Geometry check sheet. Reference: the model listing, model coordinates, mm. Face numbers are marked on the shaded views. A direction names the side the tool comes from. Give positions to 0.01 mm unless a question says otherwise; leave off trailing zeros. Write each loop counter-clockwise with the first axis right and the second up, starting at its lowest first coordinate (ties: lowest second). Pieces come first, ordered by that corner, then holes. Notation, with made-up numbers: M 1,54.5 L 38,54.5 A21 ccw 38,82.5 Z; hole C 12.5,50.25 d9. An arc over 180 degrees is marked long. Write each question's results on one line, items separated by ' | '.
```python
from build123d import *

# Parameters (mm, degrees)
BOSS_EXTRU_1_DEPTH      = 3
BOSS_EXTRU_2_START      = -3
ESQUISSE2_W             = 33.166247904
ESQUISSE2_H             = 3
BOSS_EXTRU_2_DEPTH      = 10
ENL_V_MAT_EXTRU_1_DEPTH = 10
ESQUISSE4_R             = 1.5
ENL_V_MAT_EXTRU_2_DEPTH = 10
ESQUISSE5_R             = 1
ENL_V_MAT_EXTRU_3_DEPTH = 44.588989435
ENL_V_MAT_EXTRU_4_DEPTH = 45.373415465
ESQUISSE7_R             = 1.5
ENL_V_MAT_EXTRU_5_DEPTH = 45.373415465
ESQUISSE8_R             = 1
ENL_V_MAT_EXTRU_6_DEPTH = 3


with BuildPart() as part:
    # Esquisse1 → Boss.-Extru.1 (new body)
    with BuildSketch(Plane.XY):
        with BuildLine():
            Line((16.583123952, 25), (-16.583123952, 25))
            ThreePointArc((-16.583123952, 25), (-14.186371655, -26.433820369), (30, 0))
            ThreePointArc((30, 0), (26.433820369, 14.186371655), (16.583123952, 25))
        make_face()
    extrude(amount=BOSS_EXTRU_1_DEPTH)

    # Esquisse2 → Boss.-Extru.2 (add)
    with BuildSketch(Plane(origin=(0, 0, 0), x_dir=(-1, 0, 0), z_dir=(0, 0, -1)).offset(BOSS_EXTRU_2_START)):
        with Locations((0, 23.5)):
            Rectangle(ESQUISSE2_W, ESQUISSE2_H)
    extrude(amount=-BOSS_EXTRU_2_DEPTH)

    # Esquisse3 → Enlèv. mat.-Extru.1 (cut)
    with BuildSketch(Plane(origin=(0, 25, 0), x_dir=(1, 0, 0), z_dir=(0, 1, 0))):
        with BuildLine():
            Line((13.498123952, -13), (16.583123952, -13))
            Line((16.583123952, -13), (16.583123952, -10.204860243))
            ThreePointArc((16.583123952, -10.204860243), (15.105407222, -11.673931516), (13.498123952, -13))
        make_face()
        with BuildLine():
            Line((-16.583123952, -10.208951902), (-16.583123952, -13))
            Line((-16.583123952, -13), (-13.501876048, -13))
            ThreePointArc((-13.501876048, -13), (-15.107102171, -11.675795147), (-16.583123952, -10.208951902))
        make_face()
    extrude(amount=-ENL_V_MAT_EXTRU_1_DEPTH, mode=Mode.SUBTRACT)

    # Esquisse4 → Enlèv. mat.-Extru.2 (cut)
    with BuildSketch(Plane.XZ.offset(-22)):
        with Locations(Location((-9.833123952, 7, 0), (0, 0, 270))):
            Circle(ESQUISSE4_R)
        with Locations(Location((9.833123952, 7, 0), (0, 0, 90))):
            Circle(ESQUISSE4_R)
    extrude(amount=-ENL_V_MAT_EXTRU_2_DEPTH, mode=Mode.SUBTRACT)

    # Esquisse5 → Enlèv. mat.-Extru.3 (cut, through all)
    with BuildSketch(Plane.XY.offset(3)):
        with Locations((10, -18.075)):
            Circle(ESQUISSE5_R)
        with Locations((10, 9.325)):
            Circle(ESQUISSE5_R)
    extrude(amount=-ENL_V_MAT_EXTRU_3_DEPTH, mode=Mode.SUBTRACT)

    # Esquisse6 → Enlèv. mat.-Extru.4 (cut, through all)
    with BuildSketch(Plane(origin=(0, 0, 0), x_dir=(-1, 0, 0), z_dir=(0, 0, -1))):
        with BuildLine():
            ThreePointArc((-12.628743756, -5.29279902), (-12.804806967, -4.79174357), (-13.182765939, -4.418645952))
            ThreePointArc((-13.182765939, -4.418645952), (-10, 6.82), (-6.817234061, -4.418645952))
            ThreePointArc((-6.817234061, -4.418645952), (-7.195193033, -4.79174357), (-7.371256244, -5.29279902))
            ThreePointArc((-7.371256244, -5.29279902), (-10, -7.645), (-12.628743756, -5.29279902))
        make_face()
    extrude(amount=-ENL_V_MAT_EXTRU_4_DEPTH, mode=Mode.SUBTRACT)

    # Esquisse7 → Enlèv. mat.-Extru.5 (cut, through all)
    with BuildSketch(Plane(origin=(0, 0, 0), x_dir=(-1, 0, 0), z_dir=(0, 0, -1))):
        with Locations((7.92, 0.75)):
            Circle(ESQUISSE7_R)
    extrude(amount=-ENL_V_MAT_EXTRU_5_DEPTH, mode=Mode.SUBTRACT)

    # Esquisse8 → Enlèv. mat.-Extru.6 (cut)
    with BuildSketch(Plane(origin=(0, 0, 0), x_dir=(-1, 0, 0), z_dir=(0, 0, -1))):
        with Locations((-8.25, -15)):
            Circle(ESQUISSE8_R)
        with Locations((5.08, -15)):
            Circle(ESQUISSE8_R)
    extrude(amount=-ENL_V_MAT_EXTRU_6_DEPTH, mode=Mode.SUBTRACT)


solid = part.part
```
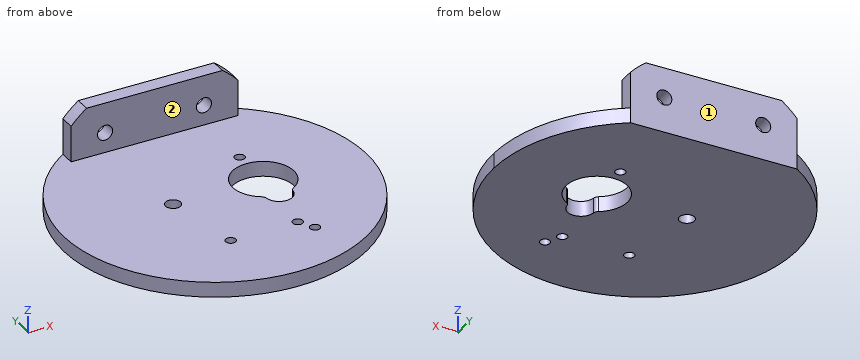
Q1. Section check D-D (y = 20). Enter the section's corners in (x, z).
Answer key:
outline: M -22.36,0 L 22.36,0 L 22.36,3 L -22.36,3 Z
Q2. Section check A-A (z = 7). Enter the section's corners in (x, y), then the cut area to 3 significant figures.
Answer key:
outline: M -16.58,22 L -11.33,22 L -11.33,25 L -16.58,25 Z; M -8.33,22 L 8.33,22 L 8.33,25 L -8.33,25 Z; M 11.33,22 L 16.58,22 L 16.58,25 L 11.33,25 Z | area: 81.5 mm2
Q3. Depth check by flat-ended pin: P1, Ø1.6, axis at x = -5.08, y = -15, coming from the -Z side; P2, Ø8, axis at x = -15.5, y = 7.5, coming from the +Z side; P3, Ø12, axis at x = -9.5, y = 6.5, coming from the -Z side; P4, Ø3.5, axis at y = 24, z = 5.5, coming from the -X side. Enter the tip coordinate at first touch or a pass-through.
Answer key:
P1: passes through | P2: stops at z = 3 | P3: stops at z = 0 | P4: stops at x = -16.58
Q4. Material ranges on probe 1 along X at (y, z) = (24, 7); probe 2 along X at (y, z) = (1, 2.25); probe 3 along Z at (x, y) = (26, 7.5), recorded low to high. Write a range as [from, to].
Answer key:
probe 1: x = [-16.58, -11.33], [-8.33, 8.33], [11.33, 16.58] | probe 2: x = [-29.98, -9.4], [-6.44, 3.94], [16.06, 29.98] | probe 3: z = [0, 3]
Q5. Section check B-B (x = -5.08). Enter the section's corners in (y, z).
Answer key:
outline: M -29.57,0 L -16,0 L -16,3 L -29.57,3 Z; M -14,0 L 25,0 L 25,13 L 22,13 L 22,3 L -14,3 Z
Q6. Section check C-C (y = 0.75). Enter the section's corners in (x, z).
Answer key:
outline: M -29.99,0 L -9.42,0 L -9.42,3 L -29.99,3 Z; M -6.42,0 L 3.93,0 L 3.93,3 L -6.42,3 Z; M 16.07,0 L 29.99,0 L 29.99,3 L 16.07,3 Z
Q7. Access from +Z, -Z, +X, -X, +Y, -Y to the whole of each face (thin tool, end or side, straight path). Record for the marked faces 1 and 2.
Answer key:
face 1: +Z, -Z, +X, -X, +Y | face 2: +Z, +X, -X, -Y
